Design review of the part built by this model. Coordinates are the model's own, in mm. Face numbers are marked on the shaded views. A direction names the side the tool comes from. Give positions to 0.01 mm unless a question says otherwise; leave off trailing zeros. Loops run counter-clockwise (first coordinate to the right, second up) from the corner with the lowest first, then second, coordinate; pieces in that order, holes last. Notation, with made-up numbers: (26.25, 9.25) -> (68.25, 9.25) arc R10 ccw to (68.25, 21.25) -> close; hole circle Ø11 at (-1.5, 66). An arc over 180 degrees is marked (long way). Use CSV: the item, a comma, the result in double quotes. Start each with the question number.
Item 1: We need section D-D (x = 8.25). State the section outline as (y, z) points, plus the area to 3 significant figures.
Item 2: We need section C-C (x = -9.5). State the section outline as (y, z) points, plus the area to 3 significant figures.
Item 3: We need section B-B (y = 2.25). State the section outline as (x, z) points, plus the area to 3 significant figures.
Item 4: We need section A-A (z = 6.3). State the section outline as (x, y) points, plus the area to 3 significant figures.
Item 5: The part is to be moulded in two halves that separate along X. For the marked faces 4, 5 and 6, say which applies: +X half, -X half, draft (parallel to the pull), parting line (faces both ways), or undercut.
Item 6: For the marked faces 1, 2 and 3, list the 3-axis set-ups (+Z, -Z, +X, -X, +Y, -Y) from which the entire face can be reached by the end or side of a thin tool; tool diameter is ignored.
Item 7: Clearance check with flat-ended pins moving along their axes: pin 1 (1 mm diameter, centred on x = 8, z = 6.5, fed in from -Y); pin 2 (3 mm diameter, centred on x = -6, z = 1.5, fed in from +Y); pin 3 (4 mm diameter, centred on x = -0.5, y = 6.5, fed in from -Z); pin 4 (3.5 mm diameter, centred on y = -1.5, z = 2, fed in from +X). State where each tip first meets the part, or that it passes through.
Item 8: Wall thickness on line 1 along X through (y, z) = (1.25, 6.3); line 2 along Y through (x, z) = (-5.25, 2.75); line 3 along Y through (x, z) = (6.75, 3): over which ranges is each line inside the solid? List them lowest first. Write a range as from..to.
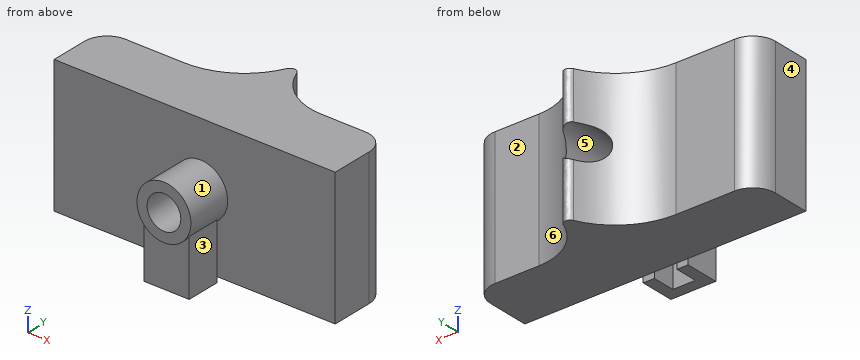
from build123d import *

# Parameters (mm, degrees)
F1_DEPTH = 12
F2_R     = 1.5
F3_DEPTH = 25
F4_R     = 0.5
F5_R     = 2
F2_R_2   = 2.4
F6_DEPTH = 4


# Not quite as in the source:
# - a feature names something its author has since deleted; it is built from what else it names


with BuildPart() as f1:
    # F0 (on Top) → F1 (new body)
    with BuildSketch(Plane.XY):
        with BuildLine():
            Line((12.5, 6.4), (6.5829587897, 6.4))
            ThreePointArc((6.5829587897, 6.4), (2.6961571623, 8.0968384564), (1.2981383552, 12.100840336))
            ThreePointArc((1.2981383552, 12.100840336), (-0.7960029052, 7.7598319357), (-5.2829587897, 6))
            Line((-5.2829587897, 6), (-12.5, 6))
            Line((-12.5, 6), (-12.5, 0.7))
            Line((-12.5, 0.7), (12.5, 0.7))
            Line((12.5, 0.7), (12.5, 6.4))
        make_face()
    extrude(amount=F1_DEPTH)

    # F2 (on face) → F3 (cut)
    with BuildSketch(Plane.XZ.offset(-0.7)):
        with Locations((0.5329587897, 6.3)):
            Circle(F2_R)
    extrude(amount=-F3_DEPTH, mode=Mode.SUBTRACT)

    # F4
    f4_edges = [f1.edges().sort_by_distance(p)[0] for p in [
        (1.298138, 12.10084, 9.795078),
        (1.298138, 12.10084, 2.504922),
    ]]
    fillet(f4_edges, radius=F4_R)

    # F5
    f5_edges = [f1.edges().sort_by_distance(p)[0] for p in [
        (-12.5, 6, 6),
        (12.5, 6.4, 6),
    ]]
    fillet(f5_edges, radius=F5_R)

    # F2 (on face) → F6 (join)
    with BuildSketch(Plane.XZ.offset(-0.7)):
        with Locations((0.5329587897, 6.3)):
            Circle(F2_R_2)
        with Locations((0.5329587897, 6.3)):
            Circle(F2_R, mode=Mode.SUBTRACT)
    extrude(amount=F6_DEPTH)

    # F0 (on Top) → F7 (join, up to the next surface of F1)
    with BuildSketch(Plane.XY):
        Polygon((-0.4670412103, 0), (-1.4670412103, 0), (-1.4670412103, -2), (-1.4670412103, -3), (2.5329587897, -3), (2.5329587897, -2), (2.5329587897, 0), (1.5329587897, 0), (1.5329587897, -2), (-0.4670412103, -2), align=None)
    extrude(until=Until.NEXT)


solid = f1.part
Results found:
1,outline,"(0.7, 0) -> (6.4, 0) -> (6.4, 12) -> (0.7, 12) -> close"
1,area,"68.4 mm²"
2,outline,"(0.7, 0) -> (6, 0) -> (6, 12) -> (0.7, 12) -> close"
2,area,"63.6 mm²"
3,outline,"(-12.5, 0) -> (12.5, 0) -> (12.5, 12) -> (-12.5, 12) -> close; hole circle Ø3 at (0.53, 6.3)"
3,area,"293 mm²"
4,outline,"(-12.5, 0.7) -> (-1.87, 0.7) -> (-1.87, -3.3) -> (-0.97, -3.3) -> (-0.97, 7.61) arc R6.6 cw to (-5.28, 6) -> (-10.5, 6) arc R2 ccw to (-12.5, 4) -> close; (2.03, -3.3) -> (2.93, -3.3) -> (2.93, 0.7) -> (12.5, 0.7) -> (12.5, 4.4) arc R2 ccw to (10.5, 6.4) -> (6.58, 6.4) arc R5.3 cw to (2.03, 8.98) -> close"
4,area,"132 mm²"
5,face 4,"-X half"
5,face 5,"undercut"
5,face 6,"+X half"
6,face 1,"none"
6,face 2,"+Z, -Z, +X, +Y"
6,face 3,"-Z, +X, -Y"
7,pin 1,"y = 0.7"
7,pin 2,"y = 6.05"
7,pin 3,"z = 0"
7,pin 4,"x = 2.53"
8,line 1,"-12.5..-0.97, 2.03..12.5"
8,line 2,"0.7..6"
8,line 3,"0.7..6.4"
